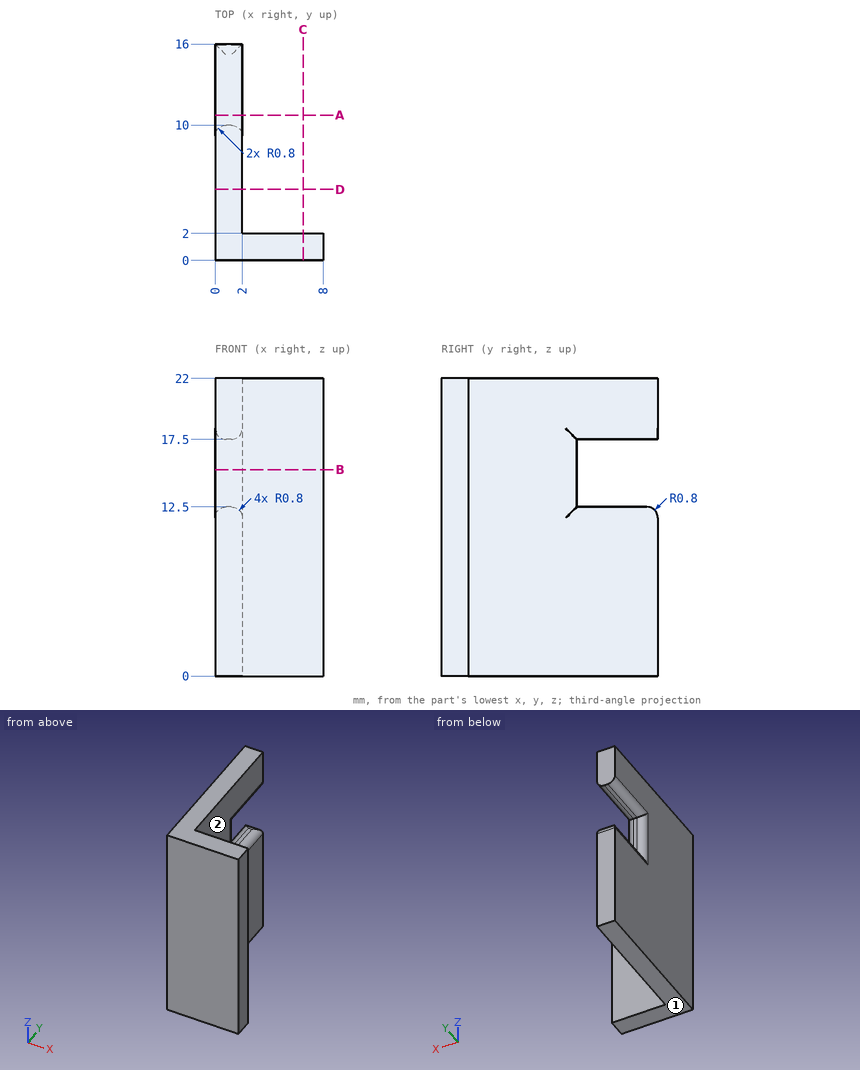
For this review, use the dimensioned drawing (mm, ordinates from the lowest corner) and the shaded views. A direction names the side the tool comes from. Coordinates: 2 decimals unless noted, no trailing zeros. Loops run counter-clockwise (first coordinate to the right, second up) from the corner with the lowest first, then second, coordinate; pieces in that order, holes last. Notation, with made-up numbers: (-23, -34.5) - (18, -34.5) arc R32 ccw to (18, -1.5) - close; hole circle Ø10 at (59, 73.5). An arc over 180 degrees is marked (long way). Use CSV: the item, a comma, the result in double quotes. Start each with the question number.
1) Tool access review of the marked faces 1 and 2: name each direction out of +Z, -Z, +X, -X, +Y, -Y from which nothing blocks a thin tool from reaching the whole face with its end or side.
2) Wall thickness on L1, parallel to X at y = 2.5, z = 4.75; L2, parallel to Z at x = 1.5, y = 13.5: over which ranges is each line inside the solid? List them lowest first. Write a range as from..to.
3) Consider section A-A on y = 10.75. Write out the cut boundary in (x, z), then the cut area to 3 significant figures.
4) For pin 1 Ø4 at (x, z) = (5, 15.5) entering from +Y; pin 2 Ø4 at (y, z) = (6, 6) entering from +X; pin 3 Ø1.5 at (x, z) = (3.5, 13.5) entering from -Y, all flat-tipped, find the tip position at first contact; note any pin that passes through.
5) Consider section B-B on z = 15.25. Write out the cut boundary in (x, y).
6) Consider section C-C on x = 6.5. Write out the cut boundary in (y, z).
Geometry says:
1,face 1,"-Z, +X, -X, +Y, -Y"
1,face 2,"+Z, -Z, +X, +Y"
2,L1,"0..2"
2,L2,"0..12.44, 17.56..22"
3,outline,"(0, 0) - (2, 0) - (2, 11.7) arc R0.8 ccw to (1.2, 12.5) - (0.8, 12.5) arc R0.8 ccw to (0, 11.7) - close; (0, 18.3) arc R0.8 ccw to (0.8, 17.5) - (1.2, 17.5) arc R0.8 ccw to (2, 18.3) - (2, 22) - (0, 22) - close"
3,area,"33.5 mm^2"
4,pin 1,"y = 2"
4,pin 2,"x = 2"
4,pin 3,"y = 0"
5,outline,"(0, 0) - (8, 0) - (8, 2) - (2, 2) - (2, 9.2) arc R0.8 ccw to (1.2, 10) - (0.8, 10) arc R0.8 ccw to (0, 9.2) - close"
6,outline,"(0, 0) - (2, 0) - (2, 22) - (0, 22) - close"
